```python
from build123d import *

# Parameters (mm, degrees)
SKETCH1_R           = 175
SKETCH1_R_2         = 160
BOSS_EXTRUDE1_DEPTH = 1.5
AXIS_GAP_DEPTH      = 248.49191906
AXIS_GAP_DEPTH_BACK = 248.49191906
SKETCH2_W           = 32.609126468
SKETCH2_H           = 20


with BuildPart() as part:
    # Sketch1 → Boss-Extrude1 (new, symmetric)
    with BuildSketch(Plane(origin=(0, 0, 0), x_dir=(1, 0, 0), z_dir=(0, 1, 0))):
        with Locations(Location((0, 0, 0), (0, 0, 270))):
            Circle(SKETCH1_R)
        with Locations(Location((0, 0, 0), (0, 0, 270))):
            Circle(SKETCH1_R_2, mode=Mode.SUBTRACT)
    extrude(amount=BOSS_EXTRUDE1_DEPTH, both=True)

    # Sketch2 → axis gap (cut, two sides: drawn at the far end of the back side and taken through both)
    with BuildSketch(Plane(origin=(0, 0, 0), x_dir=(1, 0, 0), z_dir=(0, 1, 0)).offset(-AXIS_GAP_DEPTH_BACK)):
        with Locations((167.5, 0)):
            Rectangle(SKETCH2_W, SKETCH2_H)
    extrude(amount=AXIS_GAP_DEPTH + AXIS_GAP_DEPTH_BACK, mode=Mode.SUBTRACT)


solid = part.part
```
CAD build for the part. Positions are in the model's coordinates, mm. Coordinates: 2 decimals unless noted, no trailing zeros. Order: outer loops, then holes, each group sorted by start corner. A loop starts at its lowest first (then second) coordinate and runs counter-clockwise, first axis right, second up. Notation, with made-up numbers: M 40,52 L 58,52 A23 ccw 58,67 Z; hole C -1,23.5 d11. An arc over 180 degrees is marked long. Write each question's results on one line, items separated by ' | '. Start each with the question number.
Q1. Flat gauge pins, fed straight in: P1, Ø1, axis at x = 15.5, y = -1, coming from the -Z side; P2, Ø1.5, axis at y = 0, z = -81.5, coming from the +X side. Where does each tip first touch, or does it go through?
Q2. Cut at D-D (y = -1.05). List the corners of the cut face in (x, z), then the cut area to 3 significant figures.
Q3. Drill centre lines: probe 1 along Z at (x, y) = (0, -0.8); probe 2 along Z at (x, y) = (4.5, -1.3); probe 3 along X at (y, z) = (-0.3, 0). Where is each one in solid material? Low to high. Write a range as from..to.
Q4. Cut at A-A (x = -88). List the corners of the cut face in (y, z).
Q5. Cut at C-C (x = 11.5). List the corners of the cut face in (y, z).
Q6. Cut at B-B (z = 0). List the corners of the cut face in (x, y).
Found:
1) P1: z = -174.36 | P2: x = 155.26
2) outline: M 159.69,-10 A160 cw long 159.69,10 L 174.71,10 A175 ccw long 174.71,-10 Z | area: 15,500 mm²
3) probe 1: -175..-160, 160..175 | probe 2: -174.94..-159.94, 159.94..174.94 | probe 3: -175..-160
4) outline: M -1.5,-151.26 L 1.5,-151.26 L 1.5,-133.63 L -1.5,-133.63 Z; M -1.5,133.63 L 1.5,133.63 L 1.5,151.26 L -1.5,151.26 Z
5) outline: M -1.5,-174.62 L 1.5,-174.62 L 1.5,-159.59 L -1.5,-159.59 Z; M -1.5,159.59 L 1.5,159.59 L 1.5,174.62 L -1.5,174.62 Z
6) outline: M -175,-1.5 L -160,-1.5 L -160,1.5 L -175,1.5 Z
